from build123d import *

# Parameters (mm, degrees)
SKETCH1_W           = 9
SKETCH1_H           = 20
BOSS_EXTRUDE1_DEPTH = 117.5
SKETCH3_R           = 3
CUT_EXTRUDE2_DEPTH  = 21


with BuildPart() as part:
    # Sketch1 → Boss-Extrude1 (new body, symmetric)
    with BuildSketch(Plane.XY):
        Rectangle(SKETCH1_W, SKETCH1_H)
    extrude(amount=BOSS_EXTRUDE1_DEPTH, both=True)

    # Sketch3 → Cut-Extrude2 (cut, through all)
    with BuildSketch(Plane(origin=(0, 10, 0), x_dir=(1, 0, 0), z_dir=(0, 1, 0))):
        with Locations((0, -107.5)):
            Circle(SKETCH3_R)
    cut_extrude2 = extrude(amount=-CUT_EXTRUDE2_DEPTH, mode=Mode.SUBTRACT)

    # Mirror2: Cut-Extrude2 across plane
    add(cut_extrude2.mirror(Plane.XY), mode=Mode.SUBTRACT)


solid = part.part
The model under review builds one solid part; all positions refer to its coordinate system, in mm. Round coordinates to 2 decimals unless told otherwise and drop trailing zeros. Write each loop counter-clockwise with the first axis right and the second up, starting at its lowest first coordinate (ties: lowest second). Pieces come first, ordered by that corner, then holes. Notation, with made-up numbers: M 86,81.25 L 103,81.25 A30 cw 103,103.25 Z; hole C -15.75,-11.75 d2. An arc over 180 degrees is marked long. Use a Markdown table: item, result. Add a question column.
Q1. We need section C-C, the plane y = -3.5. State the section outline as (x, z) points.
Q2. We need section A-A, the plane x = 0. State the section outline as (y, z) points, plus the area to 3 significant figures.
Q3. We need section B-B, the plane z = 107.5. State the section outline as (x, y) points.
Q4. The part is to be moulded in two halves that separate along Z. For faces 1 (the face through (0, 0, 117.5)), 2 (the face through (-0.65, 0.14, 110.43)), 3 (the face through (0, -10, 2)), say which applies: pulls with the +Z half, pulls with the -Z half, needs draft (parallel to the pull), parting line crosses it, or undercut.
Q5. To check wall thickness, follow line 1 (Z direction, x = -0.5, y = -6.75); line 2 (Z direction, x = 0.75, y = -3); line 3 (X direction, y = -4.75, z = 107.5). State the ranges of each line that lie inside material, in increasing order.
Findings below:
| question | item | result |
|---|---|---|
| 1 | outline | M -4.5,-117.5 L 4.5,-117.5 L 4.5,117.5 L -4.5,117.5 Z; hole C 0,-107.5 d6; hole C 0,107.5 d6 |
| 2 | outline | M -10,-117.5 L 10,-117.5 L 10,-110.5 L -10,-110.5 Z; M -10,-104.5 L 10,-104.5 L 10,104.5 L -10,104.5 Z; M -10,110.5 L 10,110.5 L 10,117.5 L -10,117.5 Z |
| 2 | area | 4,460 mm² |
| 3 | outline | M -4.5,-10 L -3,-10 L -3,10 L -4.5,10 Z; M 3,-10 L 4.5,-10 L 4.5,10 L 3,10 Z |
| 4 | face 1 | pulls with the +Z half |
| 4 | face 2 | undercut |
| 4 | face 3 | needs draft |
| 5 | line 1 | z = -117.5 to -110.46, -104.54 to 104.54, 110.46 to 117.5 |
| 5 | line 2 | z = -117.5 to -110.4, -104.6 to 104.6, 110.4 to 117.5 |
| 5 | line 3 | x = -4.5 to -3, 3 to 4.5 |
